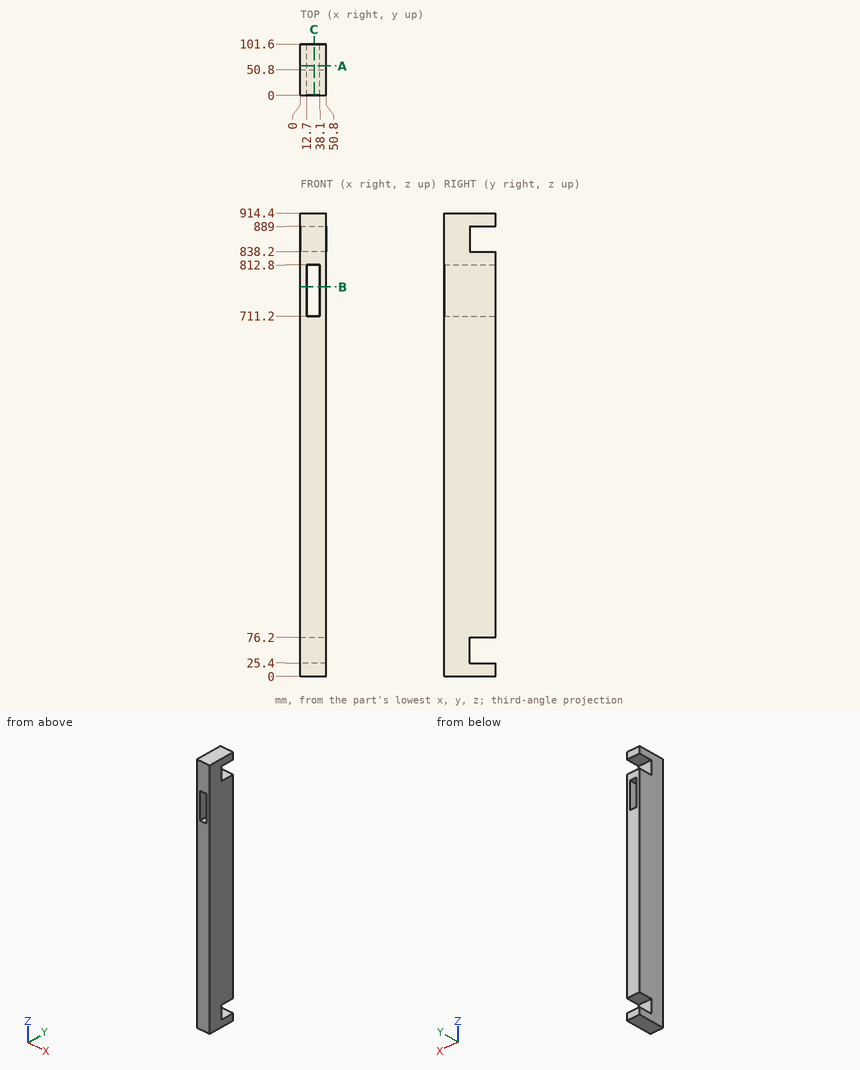
Source: three-view drawing plus pictorial views. Frame: mm from the lowest corner of the part. Coordinates: 2 decimals unless noted, no trailing zeros. Order: outer loops, then holes, each group sorted by start corner. A loop starts at its lowest first (then second) coordinate and runs counter-clockwise, first axis right, second up. Notation, with made-up numbers: M -16.5,38 L 8.5,38 A29 ccw 8.5,66 Z; hole C -14.75,17.5 d4. An arc over 180 degrees is marked long. Write each question's results on one line, items separated by ' | '. Start each with the question number.
1. Material intervals for L1, parallel to Z at x = 28, y = 58; L2, parallel to Z at x = 41, y = 59; L3, parallel to Z at x = 33, y = 20, sorted ascending.
2. Section C-C, the plane x = 27. Return the cut outline in (y, z).
3. Section A-A, the plane y = 58.5. Return the cut outline in (x, z), then the cut area to 3 significant figures.
4. Section B-B, the plane z = 769. Return the cut outline in (x, y).
Solution:
1) L1: 0 to 25.4, 76.2 to 711.2, 812.8 to 838.2, 889 to 914.4 | L2: 0 to 25.4, 76.2 to 838.2, 889 to 914.4 | L3: 0 to 711.2, 812.8 to 914.4
2) outline: M 0,0 L 101.6,0 L 101.6,25.4 L 50.8,25.4 L 50.8,76.2 L 101.6,76.2 L 101.6,711.2 L 0,711.2 Z; M 0,812.8 L 101.6,812.8 L 101.6,838.2 L 50.8,838.2 L 50.8,889 L 101.6,889 L 101.6,914.4 L 0,914.4 Z
3) outline: M 0,0 L 50.8,0 L 50.8,25.4 L 0,25.4 Z; M 0,76.2 L 50.8,76.2 L 50.8,838.2 L 0,838.2 Z; M 0,889 L 50.8,889 L 50.8,914.4 L 0,914.4 Z; hole M 12.7,711.2 L 38.1,711.2 L 38.1,812.8 L 12.7,812.8 Z | area: 38,700 mm²
4) outline: M 0,0 L 12.7,0 L 12.7,101.6 L 0,101.6 Z; M 38.1,0 L 50.8,0 L 50.8,101.6 L 38.1,101.6 Z
